Work out the finished part from the listing and answer in its coordinate system (mm). A direction names the side the tool comes from. Coordinates: 2 decimals unless noted, no trailing zeros. Write each loop counter-clockwise with the first axis right and the second up, starting at its lowest first coordinate (ties: lowest second). Pieces come first, ordered by that corner, then holes. Notation, with made-up numbers: (74.25, -6) - (111.25, -6) arc R19 cw to (111.25, 13) - close; hole circle Ø5 at (19.5, -40). An arc over 180 degrees is marked (long way). Use one line per item in the form item = value. Start each with the question number.
Item 1: A cutting plane is placed at A-A (z = -13). Write down the section's boundary in (x, y), then the cut area to 3 significant figures.
Item 2: For faces 5 (the flat face through (-1, 0, 24)), 6 (the flat face through (-24, 93, 23)), 7 (the cylindrical face through (-108, 74, 24)), determine the directions among +Z, -Z, +X, -X, +Y, -Y from which every point of the face is accessible in a straight line to the end or side of a thin tool.
Item 3: Determine the mould class of faces 1 (the cylindrical face through (119, 76, 23)), 2 (the cylindrical face through (-109, 52, 24)), 3 (the flat face through (-1, 154, 24)), 4 (the cylindrical face through (108, 116, 24)) for opening direction Y: released by +Y, released by -Y, zero draft, split by the parting line, or undercut.
Item 4: Consider probe 1 along Y at (x, z) = (-56, 23.5); probe 2 along X at (y, z) = (75, 4); probe 3 along Z at (x, y) = (-79.5, 127). Determine where each line is inside the solid, lowest interval first.
Item 5: A cutting plane is placed at C-C (y = 60). Write down the section's boundary in (x, z).
Item 6: A cutting plane is placed at D-D (x = -5). Write down the section's boundary in (y, z).
Item 7: Given pin 1 (1.6 mm diameter, centred on x = 118.5, y = 52, fed in from -Z); pin 2 (2 mm diameter, centred on y = 130.5, z = 23.5, fed in from -X); pin 3 (0.6 mm diameter, centred on y = 63.5, z = 24, fed in from +X), each flat-ended and moving along its own axis, determine where each tip first touches the part or whether it passes through.
Item 8: A cutting plane is placed at B-B (x = 51). Write down the section's boundary in (y, z), then the cut area to 3 significant figures.
from build123d import *

# Parameters (mm, degrees)
PAD001_DEPTH    = 154
POCKET_DEPTH    = 5
POCKET001_DEPTH = 5


with BuildPart() as part:
    # Sketch001 (on XZ_Plane001 of Origin002) → Pad001 (new body)
    with BuildSketch(Plane.XZ):
        with BuildLine():
            Line((-120, 20), (-120, -20))
            ThreePointArc((-120, -20), (-118.535534, -23.535534), (-115, -25))
            Line((-115, -25), (115, -25))
            ThreePointArc((115, -25), (118.535534, -23.535534), (120, -20))
            Line((120, -20), (120, 20))
            ThreePointArc((120, 20), (118.535534, 23.535534), (115, 25))
            Line((115, 25), (-115, 25))
            ThreePointArc((-115, 25), (-118.535534, 23.535534), (-120, 20))
        make_face()
        with BuildLine():
            Line((-118, 20), (-118, -20))
            ThreePointArc((-118, -20), (-117.12132, -22.12132), (-115, -23))
            Line((-115, -23), (115, -23))
            ThreePointArc((115, -23), (117.12132, -22.12132), (118, -20))
            Line((118, -20), (118, 20))
            ThreePointArc((118, 20), (117.12132, 22.12132), (115, 23))
            Line((115, 23), (-115, 23))
            ThreePointArc((-115, 23), (-117.12132, 22.12132), (-118, 20))
        make_face(mode=Mode.SUBTRACT)
    extrude(amount=-PAD001_DEPTH)

    # Sketch003 (on Face7 of Pad001) → Pocket (cut)
    with BuildSketch(Plane.XY.offset(25)):
        with BuildLine():
            Line((106, 75), (4, 75))
            ThreePointArc((4, 75), (1.171573, 73.828427), (0, 71))
            Line((0, 71), (0, 9))
            ThreePointArc((0, 9), (1.171573, 6.171573), (4, 5))
            Line((4, 5), (106, 5))
            ThreePointArc((106, 5), (108.828427, 6.171573), (110, 9))
            Line((110, 9), (110, 71))
            ThreePointArc((110, 71), (108.828427, 73.828427), (106, 75))
        make_face()
        with BuildLine():
            Line((-110, 70), (-110, 55))
            ThreePointArc((-110, 55), (-108.535534, 51.464466), (-105, 50))
            Line((-105, 50), (-15, 50))
            ThreePointArc((-15, 50), (-11.464466, 51.464466), (-10, 55))
            Line((-10, 55), (-10, 70))
            ThreePointArc((-10, 70), (-11.464466, 73.535534), (-15, 75))
            Line((-15, 75), (-105, 75))
            ThreePointArc((-105, 75), (-108.535534, 73.535534), (-110, 70))
        make_face()
        with BuildLine():
            Line((0, 135), (0, 120))
            ThreePointArc((0, 120), (1.464466, 116.464466), (5, 115))
            Line((5, 115), (105, 115))
            ThreePointArc((105, 115), (108.535534, 116.464466), (110, 120))
            Line((110, 120), (110, 135))
            ThreePointArc((110, 135), (108.535534, 138.535534), (105, 140))
            Line((105, 140), (5, 140))
            ThreePointArc((5, 140), (1.464466, 138.535534), (0, 135))
        make_face()
    extrude(amount=-POCKET_DEPTH, mode=Mode.SUBTRACT)

    # Sketch004 (on Face9 of Pocket) → Pocket001 (cut)
    with BuildSketch(Plane.YZ.offset(120)):
        with BuildLine():
            Line((45, 3), (45, -3))
            ThreePointArc((45, -3), (45.585786, -4.414214), (47, -5))
            Line((47, -5), (65, -5))
            ThreePointArc((65, -5), (66.414214, -4.414214), (67, -3))
            Line((67, -3), (67, 3))
            ThreePointArc((67, 3), (66.414214, 4.414214), (65, 5))
            Line((65, 5), (47, 5))
            ThreePointArc((47, 5), (45.585786, 4.414214), (45, 3))
        make_face()
    extrude(amount=-POCKET001_DEPTH, mode=Mode.SUBTRACT)


solid = part.part
Answer:
q1.outline = (-120, 0) - (-118, 0) - (-118, 154) - (-120, 154) - close; (118, 0) - (120, 0) - (120, 154) - (118, 154) - close
q1.area = 616 mm²
q2.face_5 = +Z, -Z, +X, -X, -Y
q2.face_6 = +Y, -Y
q2.face_7 = +Z
q3.face_1 = zero draft
q3.face_2 = undercut
q3.face_3 = released by +Y
q3.face_4 = undercut
q4.probe_1 = 0 to 50, 75 to 154
q4.probe_2 = -120 to -118, 118 to 120
q4.probe_3 = -25 to -23, 23 to 25
q5.outline = (-120, -20) arc R5 ccw to (-115, -25) - (115, -25) arc R5 ccw to (120, -20) - (120, -5) - (118, -5) - (118, -20) arc R3 cw to (115, -23) - (-115, -23) arc R3 cw to (-118, -20) - (-118, 20) arc R3 cw to (-115, 23) - (-110, 23) - (-110, 25) - (-115, 25) arc R5 ccw to (-120, 20) - close; (-10, 23) - (0, 23) - (0, 25) - (-10, 25) - close; (110, 23) - (115, 23) arc R3 cw to (118, 20) - (118, 5) - (120, 5) - (120, 20) arc R5 ccw to (115, 25) - (110, 25) - close
q6.outline = (0, -25) - (154, -25) - (154, -23) - (0, -23) - close; (0, 23) - (154, 23) - (154, 25) - (0, 25) - close
q7.pin_1 = -24.21
q7.pin_2 = -119.33
q7.pin_3 = 118.36
q8.outline = (0, -25) - (154, -25) - (154, -23) - (0, -23) - close; (0, 23) - (5, 23) - (5, 25) - (0, 25) - close; (75, 23) - (115, 23) - (115, 25) - (75, 25) - close; (140, 23) - (154, 23) - (154, 25) - (140, 25) - close
q8.area = 426 mm²
